Autodesk Inventor part; units mm, degrees
ref_plane "YZ Plane" through (0, 0, 0) normal (1, 0, 0) x (0, 1, 0)
ref_plane "XZ Plane" through (0, 0, 0) normal (0, 1, 0) x (-1, 0, 0)
ref_plane "XY Plane" through (0, 0, 0) normal (0, 0, 1) x (1, 0, 0)
sketch "Skizze1" plane through (0, 0, 0) normal (0, 0, 1) x (1, 0, 0)
  line L0 (-199, -212.5) -> (199, -212.5)
  line L1 (199, -212.5) -> (199, 212.5)
  line L2 (199, 212.5) -> (-199, 212.5)
  line L3 (-199, 212.5) -> (-199, -212.5)
  line L4 (-199, -212.5) -> (199, 212.5) construction
  line L5 (199, -212.5) -> (-199, 212.5) construction
  line L6 (182, -195.5) -> (-182, -195.5)
  line L7 (-182, -195.5) -> (-182, 204.5)
  line L8 (-182, 204.5) -> (182, 204.5)
  line L9 (182, 204.5) -> (182, -195.5)
  line L10 (182, -195.5) -> (-182, 204.5) construction
  line L11 (-182, -195.5) -> (182, 204.5) construction
  point P0 (0, 0)
  dimension "d0" = 398
  dimension "d1" = 425
  dimension "d5" = 17
  dimension "d8" = 17
  dimension "d9" = 17
  dimension "d10" = 8
extrude "Extrusion1" add sketch "Skizze1" along normal blind 15 contours L3 L2 L1 L0 | L6 L7 L8 L9
extrude "Extrusion2" add sketch "Skizze1" against normal blind 6 contours L6 L7 L8 L9
equation "\"d0\" = case_width - 2 * gap_air"
equation "\"d2\" = inner_thickness"
equation "\"d6\" = mdf_thickness"
equation "\"kg_thickness\" = 4.9"
equation "\"ht_thickness\" = 1.9"
equation "\"case_thickness\" = 18"
equation "\"inner_thickness\" = 15"
equation "\"gap_fit\" = 0.1"
equation "\"gap_slide\" = 0.2"
equation "\"gap_air\" = 1"
equation "\"bore_diameter\" = 73"
equation "\"mdf_thickness\" = 6"
equation "\"tape_width\" = 15"
equation "\"tape_thickness\" = 3"
equation "\"inner_depth\" = 255"
properties part number "Front_Staubfach"
Input: part model. Units: mm. Frame: model coordinates. Give positions to 0.01 mm unless a question says otherwise; leave off trailing zeros. Loops run counter-clockwise (first coordinate to the right, second up) from the corner with the lowest first, then second, coordinate; pieces in that order, holes last. Notation, with made-up numbers: M 48.25,18 L 78.25,18 A24 cw 78.25,46 Z; hole C -24.75,-33.75 d6. An arc over 180 degrees is marked long. Use one line per item in the form item = value.
1. Section query A-A, the plane x = 60.5. Return the cut outline in (y, z).
Numbers:
outline = M -212.5,0 L -195.5,0 L -195.5,-6 L 204.5,-6 L 204.5,0 L 212.5,0 L 212.5,15 L -212.5,15 Z
2. Line query: L1, parallel to X at y = -147, z = -3.25; L2, parallel to Y at x = 140, z = -1.75. Output: solid intervals per line, ascending.
Numbers:
L1 = -182 to 182
L2 = -195.5 to 204.5
3. Section query B-B, the plane y = 66.5. Return the cut outline in (x, z).
Numbers:
outline = M -199,0 L -182,0 L -182,-6 L 182,-6 L 182,0 L 199,0 L 199,15 L -199,15 Z
4. First-contact query: pin 1 (1.8 mm diameter, centred on y = -31.5, z = -2, fed in from -X); pin 2 (3 mm diameter, centred on x = 33, z = -3.5, fed in from -Y). Flat tips, straight axial feed; report the tip coordinate or a pass-through.
Numbers:
pin_1 = -182
pin_2 = -195.5
